```python
from build123d import *

# Parameters (mm, degrees)
SKETCH1_R           = 15
BOSS_EXTRUDE1_DEPTH = 22
SCALE1_SCALE        = 0.1


with BuildPart() as part:
    # Sketch1 → Boss-Extrude1 (new body)
    with BuildSketch(Plane(origin=(0, 0, 0), x_dir=(1, 0, 0), z_dir=(0, 1, 0))):
        Polygon((17.033110265, -5.228113471), (17.033110265, 29.771886529), (-13.277778868, 47.271886529), (-43.588668, 29.771886529), (-43.588668, -5.228113471), (-13.277778868, -22.728113471), align=None)
        with Locations((-13.277778868, 12.271886529)):
            Circle(SKETCH1_R, mode=Mode.SUBTRACT)
    extrude(amount=BOSS_EXTRUDE1_DEPTH)


with BuildPart() as part_1:
    # Scale1: scaled about (-13.277778868, 11, -12.271886529)
    add(part.part.scale(SCALE1_SCALE).moved(Location((-11.950000981, 9.9, -11.044697876))))


solid = part_1.part
```
The model under review builds one solid part; all positions refer to its coordinate system, in mm. Give positions to 0.01 mm unless a question says otherwise; leave off trailing zeros. Write each loop counter-clockwise with the first axis right and the second up, starting at its lowest first coordinate (ties: lowest second). Pieces come first, ordered by that corner, then holes.
(1) For P1, Ø3.5, axis at x = -13.28, z = -12.27, coming from the +Y side, flat-tipped, find the tip position at first contact; note if it passes through.
(2) Consider section B-B, the plane z = -11.75. Give the boundary of the cut face in (x, y).
(3) The part is to be moulded in two halves that separate along X. For faces 1 (the cylindrical face through (-12.471, 10.985, -13.537)), 2 (the flat face through (-11.783, 10.985, -9.635)), 3 (the flat face through (-16.309, 11, -12)), say which applies: released by +X, released by -X, zero draft, split by the parting line, or undercut.
(4) To check wall thickness, follow L1, parallel to Z at x = -12.25, y = 10.85; L2, parallel to X at y = 11.6, z = -13; L3, parallel to Z at x = -13, y = 10.9. State the ranges of each line that lie inside material, in increasing order.
(5) Consider section A-A, the plane x = -12.5. Give the boundary of the cut face in (y, z), and give its area (3 significant figures).
(6) Consider section C-C, the plane y = 10.8. Give the boundary of the cut face in (x, z).
(7) Consider section D-D, the plane z = -15. Give the boundary of the cut face in (x, y).
Returned:
1. P1: stops at y = 12.1
2. outline: (-16.31, 9.9) - (-14.68, 9.9) - (-14.68, 12.1) - (-16.31, 12.1) - close; (-11.87, 9.9) - (-10.25, 9.9) - (-10.25, 12.1) - (-11.87, 12.1) - close
3. face 1: undercut
3. face 2: released by +X
3. face 3: released by -X
4. L1: z = -15.18 to -13.36, -11.18 to -9.37
4. L2: x = -16.31 to -14.59, -11.97 to -10.25
4. L3: z = -15.61 to -13.75, -10.8 to -8.93
5. outline: (9.9, -15.32) - (12.1, -15.32) - (12.1, -13.55) - (9.9, -13.55) - close; (9.9, -10.99) - (12.1, -10.99) - (12.1, -9.22) - (9.9, -9.22) - close
5. area: 7.78 mm2
6. outline: (-16.31, -14.02) - (-13.28, -15.77) - (-10.25, -14.02) - (-10.25, -10.52) - (-13.28, -8.77) - (-16.31, -10.52) - close; hole circle Ø3 at (-13.28, -12.27)
7. outline: (-14.61, 9.9) - (-11.94, 9.9) - (-11.94, 12.1) - (-14.61, 12.1) - close
